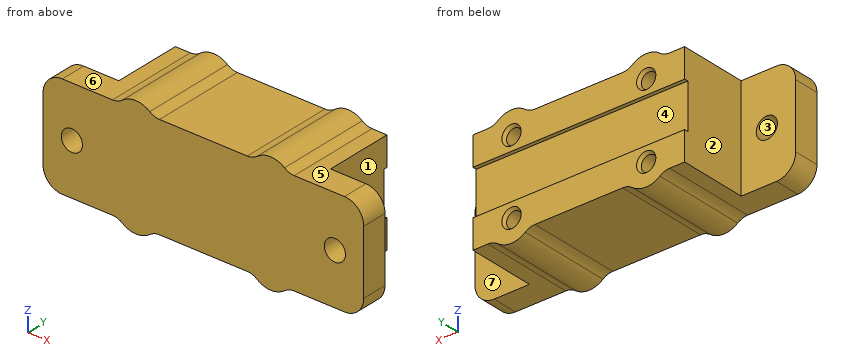
from build123d import *

# Parameters (mm, degrees)
CROQUIS1_W                = 50
CROQUIS1_H                = 16
CROQUIS1_R                = 1.65
SALIENTE_EXTRUIR1_DEPTH   = 4
CROQUIS2_W                = 33
CROQUIS2_H                = 16
SALIENTE_EXTRUIR2_DEPTH   = 10
CROQUIS3_W                = 33
CROQUIS3_H                = 4.5
SALIENTE_EXTRUIR3_DEPTH   = 0.6
CROQUIS4_R                = 1.2
CORTAR_EXTRUIR1_DEPTH     = 8
SALIENTE_EXTRUIR5_DEPTH   = 14.6
SIMETR_A2_COPY_1_DEPTH    = 14.6
REDONDEO1_R               = 3
REDONDEO2_R               = 3
REDONDEO3_R               = 3
REDONDEO4_R               = 3
CROQUIS6_R                = 1.5
CORTAR_EXTRUIR2_DEPTH     = 0.6
CORTAR_EXTRUIR2_TAPER     = 30
SIMETR_A6_COPY_1_SKETCH_R = 1.5
SIMETR_A6_COPY_1_DEPTH    = 0.6
SIMETR_A6_COPY_1_TAPER    = 30


with BuildPart() as part:
    # Croquis1 → Saliente-Extruir1 (new body)
    with BuildSketch(Plane(origin=(0, 0, 0), x_dir=(1, 0, 0), z_dir=(0, 1, 0))):
        with Locations((25, -8)):
            Rectangle(CROQUIS1_W, CROQUIS1_H)
        with Locations((4.5, -8)):
            Circle(CROQUIS1_R, mode=Mode.SUBTRACT)
        with Locations((45.5, -8)):
            Circle(CROQUIS1_R, mode=Mode.SUBTRACT)
    extrude(amount=SALIENTE_EXTRUIR1_DEPTH)

    # Croquis2 → Saliente-Extruir2 (add)
    with BuildSketch(Plane(origin=(0, 4, 0), x_dir=(1, 0, 0), z_dir=(0, 1, 0))):
        with Locations((25, -8)):
            Rectangle(CROQUIS2_W, CROQUIS2_H)
    extrude(amount=SALIENTE_EXTRUIR2_DEPTH)

    # Croquis3 → Saliente-Extruir3 (add)
    with BuildSketch(Plane(origin=(0, 14, 0), x_dir=(1, 0, 0), z_dir=(0, 1, 0))):
        with Locations((25, -2.25)):
            Rectangle(CROQUIS3_W, CROQUIS3_H)
        with Locations((25, -13.75)):
            Rectangle(CROQUIS3_W, CROQUIS3_H)
    extrude(amount=SALIENTE_EXTRUIR3_DEPTH)

    # Croquis4 → Cortar-Extruir1 (cut)
    with BuildSketch(Plane(origin=(0, 14.6, 0), x_dir=(1, 0, 0), z_dir=(0, 1, 0))):
        with Locations((14.5, -13.75)):
            Circle(CROQUIS4_R)
        with Locations((14.5, -2.25)):
            Circle(CROQUIS4_R)
        with Locations((35.5, -13.75)):
            Circle(CROQUIS4_R)
        with Locations((35.5, -2.25)):
            Circle(CROQUIS4_R)
    extrude(amount=-CORTAR_EXTRUIR1_DEPTH, mode=Mode.SUBTRACT)

    # Croquis5 → Saliente-Extruir5 (add)
    with BuildSketch(Plane(origin=(0, 14.6, 0), x_dir=(1, 0, 0), z_dir=(0, 1, 0))):
        with BuildLine():
            Line((18.165719575, -16), (10.834280425, -16))
            ThreePointArc((10.834280425, -16), (11.641151956, -16.133788189), (12.361663581, -16.520833333))
            ThreePointArc((12.361663581, -16.520833333), (14.5, -17.25), (16.638336419, -16.520833333))
            ThreePointArc((16.638336419, -16.520833333), (17.358848044, -16.133788189), (18.165719575, -16))
        make_face()
    saliente_extruir5 = extrude(amount=-SALIENTE_EXTRUIR5_DEPTH)

    # Simetría1: Saliente-Extruir5 across plane
    add(saliente_extruir5.mirror(Plane.ZY.offset(-25)))

    # Simetría2: Saliente-Extruir5 across plane
    add(saliente_extruir5.mirror(Plane.XY.offset(8)))

    # Simetría2 copy 1 sketch → Simetría2 copy 1 (add)
    with BuildSketch(Plane(origin=(50, 14.6, 16), x_dir=(-1, 0, 0), z_dir=(0, 1, 0))):
        with BuildLine():
            Line((18.165719575, -16), (10.834280425, -16))
            ThreePointArc((10.834280425, -16), (11.641151956, -16.133788189), (12.361663581, -16.520833333))
            ThreePointArc((12.361663581, -16.520833333), (14.5, -17.25), (16.638336419, -16.520833333))
            ThreePointArc((16.638336419, -16.520833333), (17.358848044, -16.133788189), (18.165719575, -16))
        make_face()
    extrude(amount=-SIMETR_A2_COPY_1_DEPTH)

    # Redondeo1
    redondeo1_edges = [part.edges().sort_by_distance(p)[0] for p in [
        (0, 2, 16),
    ]]
    fillet(redondeo1_edges, radius=REDONDEO1_R)

    # Redondeo2
    redondeo2_edges = [part.edges().sort_by_distance(p)[0] for p in [
        (0, 2, 0),
    ]]
    fillet(redondeo2_edges, radius=REDONDEO2_R)

    # Redondeo3
    redondeo3_edges = [part.edges().sort_by_distance(p)[0] for p in [
        (50, 2, 0),
    ]]
    fillet(redondeo3_edges, radius=REDONDEO3_R)

    # Redondeo4
    redondeo4_edges = [part.edges().sort_by_distance(p)[0] for p in [
        (50, 2, 16),
    ]]
    fillet(redondeo4_edges, radius=REDONDEO4_R)

    # Croquis6 → Cortar-Extruir2 (cut)
    with BuildSketch(Plane(origin=(0, 14.6, 0), x_dir=(1, 0, 0), z_dir=(0, 1, 0))):
        with Locations((14.5, -13.75)):
            Circle(CROQUIS6_R)
    cortar_extruir2 = extrude(amount=-CORTAR_EXTRUIR2_DEPTH, taper=CORTAR_EXTRUIR2_TAPER, mode=Mode.SUBTRACT)

    # Simetría5: Cortar-Extruir2 across plane
    add(cortar_extruir2.mirror(Plane.ZY.offset(-25)), mode=Mode.SUBTRACT)

    # Simetría6: Cortar-Extruir2 across plane
    add(cortar_extruir2.mirror(Plane.XY.offset(8)), mode=Mode.SUBTRACT)

    # Simetría6 copy 1 sketch → Simetría6 copy 1 (cut)
    with BuildSketch(Plane(origin=(50, 14.6, 16), x_dir=(-1, 0, 0), z_dir=(0, 1, 0))):
        with Locations((14.5, -13.75)):
            Circle(SIMETR_A6_COPY_1_SKETCH_R)
    extrude(amount=-SIMETR_A6_COPY_1_DEPTH, taper=SIMETR_A6_COPY_1_TAPER, mode=Mode.SUBTRACT)


solid = part.part
Could you check a few things on this model? Use its own coordinates, in mm. Face numbers are marked on the shaded views. A direction names the side the tool comes from. Give positions to 0.01 mm unless a question says otherwise; leave off trailing zeros. Write each loop counter-clockwise with the first axis right and the second up, starting at its lowest first coordinate (ties: lowest second). Pieces come first, ordered by that corner, then holes. Notation, with made-up numbers: (-32, -19.75) - (3, -19.75) arc R15 cw to (3, 5.25) - close; hole circle Ø2 at (32, 40). An arc over 180 degrees is marked (long way). Use CSV: the item, a comma, the result in double quotes. Start each with the question number.
Item 1: I'm going to push flat-ended pins straight in: pin 1 (2.5 mm diameter, centred on x = 14.5, z = 14.5, fed in from +Y); pin 2 (1.9 mm diameter, centred on x = 35.5, z = 2.25, fed in from +Y); pin 3 (4 mm diameter, centred on x = 43, y = 8, fed in from +Z); pin 4 (4 mm diameter, centred on x = 6, y = 5.5, fed in from -Z). Where does each tip first touch, or does it pass through?
Item 2: I want a section at D-D, the plane y = 6. Please give me the cut outline in (x, z), then the cut area to 3 significant figures.
Item 3: I want a section at B-B, the plane z = 7.25. Please give me the cut outline in (x, y), then the cut area to 3 significant figures.
Item 4: If we mould it in two halves opening along X, with no side actions, what happens to the marked faces 1, 2, 3 and 4? For each: pulls with the +X half, pulls with the -X half, needs draft (parallel to the pull), parting line crosses it, or undercut.
Item 5: For the marked faces 5, 6 and 7, which set-ups out of +Z, -Z, +X, -X, +Y, -Y let a thin tool reach every point of the face, with its end or its side?
Item 6: If I drill on line 1 along Z through (x, y) = (35.5, 9.25); line 2 along X through (y, z) = (12.75, 13.5); line 3 along Z through (x, y) = (36.5, 11.75), over which ranges is the centre line in solid material (lowest first)?
Item 7: I want a section at A-A, the plane x = 45.5. Please give me the cut outline in (y, z), then the cut area to 3 significant figures.
Item 8: I want a section at C-C, the plane y = 2.5. Please give me the cut outline in (x, z).
Findings:
1,pin 1,"stops at y = 14.6"
1,pin 2,"stops at y = 6.6"
1,pin 3,"stops at z = 16"
1,pin 4,"stops at z = 0"
2,outline,"(8.5, 0) - (10.83, 0) arc R2.5 cw to (12.36, -0.52) arc R3.5 ccw to (16.64, -0.52) arc R2.5 cw to (18.17, 0) - (31.83, 0) arc R2.5 cw to (33.36, -0.52) arc R3.5 ccw to (37.64, -0.52) arc R2.5 cw to (39.17, 0) - (41.5, 0) - (41.5, 16) - (39.17, 16) arc R2.5 cw to (37.64, 16.52) arc R3.5 ccw to (33.36, 16.52) arc R2.5 cw to (31.83, 16) - (18.17, 16) arc R2.5 cw to (16.64, 16.52) arc R3.5 ccw to (12.36, 16.52) arc R2.5 cw to (10.83, 16) - (8.5, 16) - close"
2,area,"547 mm2"
3,outline,"(0, 0) - (3.03, 0) - (3.03, 4) - (0, 4) - close; (5.97, 0) - (44.03, 0) - (44.03, 4) - (41.5, 4) - (41.5, 14) - (8.5, 14) - (8.5, 4) - (5.97, 4) - close; (46.97, 0) - (50, 0) - (50, 4) - (46.97, 4) - close"
3,area,"506 mm2"
4,face 1,"pulls with the +X half"
4,face 2,"pulls with the -X half"
4,face 3,"undercut"
4,face 4,"needs draft"
5,face 5,"+Z, +X, +Y, -Y"
5,face 6,"+Z, -X, +Y, -Y"
5,face 7,"+Z, -Z, +X, +Y"
6,line 1,"z = -1.25 to 1.05, 3.45 to 12.55, 14.95 to 17.25"
6,line 2,"x = 8.5 to 13.33, 15.67 to 34.33, 36.67 to 41.5"
6,line 3,"z = -1.1 to 1.59, 2.91 to 13.09, 14.41 to 17.1"
7,outline,"(0, 0) - (4, 0) - (4, 6.35) - (0, 6.35) - close; (0, 9.65) - (4, 9.65) - (4, 16) - (0, 16) - close"
7,area,"50.8 mm2"
8,outline,"(0, 3) arc R3 ccw to (3, 0) - (10.83, 0) arc R2.5 cw to (12.36, -0.52) arc R3.5 ccw to (16.64, -0.52) arc R2.5 cw to (18.17, 0) - (31.83, 0) arc R2.5 cw to (33.36, -0.52) arc R3.5 ccw to (37.64, -0.52) arc R2.5 cw to (39.17, 0) - (47, 0) arc R3 ccw to (50, 3) - (50, 13) arc R3 ccw to (47, 16) - (39.17, 16) arc R2.5 cw to (37.64, 16.52) arc R3.5 ccw to (33.36, 16.52) arc R2.5 cw to (31.83, 16) - (18.17, 16) arc R2.5 cw to (16.64, 16.52) arc R3.5 ccw to (12.36, 16.52) arc R2.5 cw to (10.83, 16) - (3, 16) arc R3 ccw to (0, 13) - close; hole circle Ø3.3 at (4.5, 8); hole circle Ø3.3 at (45.5, 8)"
